Build history of the part. All positions in model axes, mm. A direction names the side the tool comes from. Give positions to 0.01 mm unless a question says otherwise; leave off trailing zeros. Loops run counter-clockwise (first coordinate to the right, second up) from the corner with the lowest first, then second, coordinate; pieces in that order, holes last. Notation, with made-up numbers: (-16.75, 65.25) - (42.25, 65.25) arc R14 ccw to (42.25, 88.25) - close; hole circle Ø5 at (29, 6). An arc over 180 degrees is marked (long way). Return JSON: item names as keys, results as strings. Group by question number.
1) Slice it at D-D (y = 20). List the corners of the cut face in (x, z).
2) Slice it at C-C (z = -8). List the corners of the cut face in (x, y), and give its area (3 significant figures).
3) Mould opens along Z. For faces 1 (the face through (0.17, 44.7, 1.29)), 2 (the face through (19, 25, -18.55)), 3 (the face through (19.515, 5.3, -2.061)), 4 (the face through (9, 50, -2)) say: released by +Z, released by -Z, zero draft, split by the parting line, or undercut.
4) Drop flat-ended pins along their axis: pin 1 (2 mm diameter, centred on y = 39.5, z = -7, fed in from -X); pin 2 (8.5 mm diameter, centred on x = 13, y = 47, fed in from +Z); pin 3 (2.5 mm diameter, centred on x = 0, z = 0, fed in from -Y); pin 4 (12 mm diameter, centred on x = 6.5, y = 45, fed in from -Z). Give the stop position or say it passes through.
5) Slice it at B-B (y = 5). List the corners of the cut face in (x, z), and give its area (3 significant figures).
6) Slice it at A-A (x = 15.5). List the corners of the cut face in (y, z).
7) 3-axis set-ups, long thin cutter, end or side, ignore diameter. For faces 5 (the face through (19, 25, -6.55)), 6 (the face through (9, 0, -2)), 7 (the face through (9, 5, -2.75)): which of +Z, -Z, +X, -X, +Y, -Y reach the whole face in a straight line?
8) Drill centre lines: probe 1 along Y at (x, z) = (2, -1.25); probe 2 along X at (y, z) = (7, -10.5). Where is each one in solid material? Low to high. Write a range as from..to.
```python
from build123d import *

# Parameters (mm, degrees)
F1_DEPTH = 50
F2_D     = 2.6
F3_W     = 28.5
F3_H     = 6.7
F3_H_2   = 3.3
F4_DEPTH = 25


with BuildPart() as f1:
    # F0 (on Front) → F1 (new body)
    with BuildSketch(Plane.XZ):
        with BuildLine():
            ThreePointArc((2.2715633383, -1.55), (1.2845232579, -2.4315632832), (0, -2.75))
            Line((0, -2.75), (18.3, -2.75))
            ThreePointArc((18.3, -2.75), (18.6535533906, -2.8964466094), (18.8, -3.25))
            Line((18.8, -3.25), (18.8, -18.55))
            Line((18.8, -18.55), (20, -18.55))
            Line((20, -18.55), (20, -3.25))
            ThreePointArc((20, -3.25), (19.502081528, -2.047918472), (18.3, -1.55))
            Line((18.3, -1.55), (2.2715633383, -1.55))
        make_face()
        with BuildLine():
            ThreePointArc((2.2715633383, -1.55), (2.6276699926, -0.8110797802), (2.75, 0))
            ThreePointArc((2.75, 0), (-1.9445436483, 1.9445436483), (0, -2.75))
            ThreePointArc((0, -2.75), (1.2845232579, -2.4315632832), (2.2715633383, -1.55))
        make_face()
    extrude(amount=-F1_DEPTH)

    # F2 (through all)
    with Locations(Plane.XZ):
        with Locations((0, 0)):
            Hole(F2_D / 2)

    # F3 (on face) → F4 (cut)
    with BuildSketch(Plane.YZ.offset(20)):
        with Locations((25, 0.1)):
            Rectangle(F3_W, F3_H)
        with Locations((25, -4.9)):
            Rectangle(F3_W, F3_H_2)
    extrude(amount=-F4_DEPTH, mode=Mode.SUBTRACT)


solid = f1.part
```
Results:
{
 "1": {"outline": "(18.8, -18.55) - (20, -18.55) - (20, -6.55) - (18.8, -6.55) - close"},
 "2": {"outline": "(18.8, 0) - (20, 0) - (20, 50) - (18.8, 50) - close", "area": "60.0 mm2"},
 "3": {"face 1": "undercut", "face 2": "released by -Z", "face 3": "released by +Z", "face 4": "zero draft"},
 "4": {"pin 1": "x = 18.8", "pin 2": "z = -1.55", "pin 3": "through", "pin 4": "z = -2.75"},
 "5": {"outline": "(0, -2.75) - (18.3, -2.75) arc R0.5 cw to (18.8, -3.25) - (18.8, -18.55) - (20, -18.55) - (20, -3.25) arc R1.7 ccw to (18.3, -1.55) - (2.27, -1.55) arc R2.75 ccw (long way) to start; hole circle Ø2.6 at (0, 0)", "area": "58.9 mm2"},
 "6": {"outline": "(0, -2.75) - (10.75, -2.75) - (10.75, -1.55) - (0, -1.55) - close; (39.25, -2.75) - (50, -2.75) - (50, -1.55) - (39.25, -1.55) - close"},
 "7": {"face 5": "+Z, +X, -X", "face 6": "+Z, -Z, +X, -X, -Y", "face 7": "-Z, -X, +Y, -Y"},
 "8": {"probe 1": "0..10.75, 39.25..50", "probe 2": "18.8..20"}
}
